Verification items for the finished model (mm, model axes). A direction names the side the tool comes from. Coordinates: 2 decimals unless noted, no trailing zeros. Write each loop counter-clockwise with the first axis right and the second up, starting at its lowest first coordinate (ties: lowest second). Pieces come first, ordered by that corner, then holes. Notation, with made-up numbers: (32, 66.5) -> (56, 66.5) arc R19 ccw to (56, 99.5) -> close; hole circle Ø6 at (10.25, 81.5). An arc over 180 degrees is marked (long way). Use a Markdown table: item, result. Add a question column.
from build123d import *

# Parameters (mm, degrees)
SKETCH022_R     = 9.7
PAD007_DEPTH    = 10
SKETCH023_R     = 9.7
PAD008_DEPTH    = 22
SKETCH024_R     = 8.35
POCKET013_DEPTH = 23
SKETCH025_R     = 8.2
POCKET014_DEPTH = 12


with BuildPart() as part:
    # Sketch022 → Pad007 (new body, symmetric)
    with BuildSketch(Plane.XZ):
        Circle(SKETCH022_R)
    extrude(amount=PAD007_DEPTH, both=True)

    # Sketch023 → Pad008 (join)
    with BuildSketch(Plane.YZ):
        Circle(SKETCH023_R)
    extrude(amount=PAD008_DEPTH)

    # Sketch024 → Pocket013 (cut)
    with BuildSketch(Plane.XZ.offset(10)):
        Circle(SKETCH024_R)
    extrude(amount=-POCKET013_DEPTH, mode=Mode.SUBTRACT)

    # Sketch025 → Pocket014 (cut)
    with BuildSketch(Plane.YZ.offset(22)):
        Circle(SKETCH025_R)
    extrude(amount=-POCKET014_DEPTH, mode=Mode.SUBTRACT)


solid = part.part
1) Cross-section at A-A on z = 0. Record the boundary of the cut face in (x, y).
2) Set-up check for faces 5 (the face through (16.08, -1.07, 8.13)), 6 (the face through (3, -10, 8)): record each of +Z, -Z, +X, -X, +Y, -Y from which the full face is reachable in a straight line by a thin tool's end or side.
3) Release check for a two-part mould opening along X. For faces 1 (the face through (10, 0, 0)), 2 (the face through (-9.69, -0.14, 0.43)), 3 (the face through (3, 10, 8)), 4 (the face through (7.964, -0.14, 2.508)) record: released by +X, released by -X, zero draft, split by the parting line, or undercut.
4) Cross-section at C-C on x = -5. Record the boundary of the cut face in (y, z), then the cut area to 3 significant figures.
5) Gauge pin test, flat ends, axial feed: pin 1 (6 mm diameter, centred on x = -5, y = 3.5, fed in from +Z); pin 2 (1 mm diameter, centred on x = 8, y = 5, fed in from -Z); pin 3 (3 mm diameter, centred on x = -2.5, y = -5.5, fed in from -Z). Record the tip position at first contact, or that the pin passes through.
6) Thickness scan on L1, parallel to Z at x = 14.75, y = 0; L2, parallel to Z at x = 3.5, y = -6.75; L3, parallel to X at y = -1.5, z = -6.5. Record the ranges inside material, lowest first.
7) Cross-section at D-D on z = 8.75. Record the boundary of the cut face in (x, y).
8) Cross-section at B-B on y = 0. Record the boundary of the cut face in (x, z), then the cut area to 3 significant figures.
Returned:
| question | item | result |
|---|---|---|
| 1 | outline | (-9.7, -10) -> (-8.35, -10) -> (-8.35, 10) -> (-9.7, 10) -> close; (8.35, -10) -> (9.7, -10) -> (9.7, -9.7) -> (22, -9.7) -> (22, -8.2) -> (10, -8.2) -> (10, 8.2) -> (22, 8.2) -> (22, 9.7) -> (9.7, 9.7) -> (9.7, 10) -> (8.35, 10) -> close |
| 2 | face 5 | +X |
| 2 | face 6 | +Z, -Z, +X, -X, -Y |
| 3 | face 1 | released by +X |
| 3 | face 2 | split by the parting line |
| 3 | face 3 | zero draft |
| 3 | face 4 | undercut |
| 4 | outline | (-10, -8.31) -> (10, -8.31) -> (10, -6.69) -> (-10, -6.69) -> close; (-10, 6.69) -> (10, 6.69) -> (10, 8.31) -> (-10, 8.31) -> close |
| 4 | area | 65.0 mm² |
| 5 | pin 1 | stops at z = 9.49 |
| 5 | pin 2 | stops at z = -8.59 |
| 5 | pin 3 | stops at z = -9.65 |
| 6 | L1 | z = -9.7 to -8.2, 8.2 to 9.7 |
| 6 | L2 | z = -9.05 to -7.58, 7.58 to 9.05 |
| 6 | L3 | x = -7.2 to -5.24, 5.24 to 10 |
| 7 | outline | (-4.19, -10) -> (4.19, -10) -> (4.19, -4.19) -> (22, -4.19) -> (22, 4.19) -> (4.19, 4.19) -> (4.19, 10) -> (-4.19, 10) -> close |
| 8 | outline | (0, -9.7) -> (22, -9.7) -> (22, -8.2) -> (10, -8.2) -> (10, 8.2) -> (22, 8.2) -> (22, 9.7) -> (0, 9.7) arc R9.7 ccw to start; hole circle Ø16.7 at (0, 0) |
| 8 | area | 159 mm² |
